Can you work these out from the model? Positions are in its coordinate system, mm. Coordinates: 2 decimals unless noted, no trailing zeros. Loops run counter-clockwise (first coordinate to the right, second up) from the corner with the lowest first, then second, coordinate; pieces in that order, holes last.
```python
from build123d import *

# Parameters (mm, degrees)
ESQUISSE1_W             = 143
ESQUISSE1_H             = 200
BOSS_EXTRU_1_DEPTH      = 6
ESQUISSE2_W             = 6
ESQUISSE2_H             = 30
ESQUISSE2_W_2           = 29
ESQUISSE2_H_2           = 6
ESQUISSE2_W_3           = 24
ENL_V_MAT_EXTRU_1_DEPTH = 6
ESQUISSE3_W             = 6
ESQUISSE3_H             = 37
BOSS_EXTRU_2_DEPTH      = 6
ESQUISSE4_W             = 36
ESQUISSE4_H             = 200
ENL_V_MAT_EXTRU_2_DEPTH = 10
ESQUISSE5_R             = 2.995
ENL_V_MAT_EXTRU_3_DEPTH = 3
ESQUISSE6_R             = 1.5
ENL_V_MAT_EXTRU_4_DEPTH = 6
ESQUISSE7_R             = 5
ENL_V_MAT_EXTRU_5_DEPTH = 10


with BuildPart() as part:
    # Esquisse1 → Boss.-Extru.1 (new body)
    with BuildSketch(Plane.XY):
        with Locations((-71.5, 100)):
            Rectangle(ESQUISSE1_W, ESQUISSE1_H)
    extrude(amount=BOSS_EXTRU_1_DEPTH)

    # Esquisse2 → Enlèv. mat.-Extru.1 (cut)
    with BuildSketch(Plane(origin=(0, 0, 0), x_dir=(-1, 0, 0), z_dir=(0, 0, -1))):
        with Locations((3, 65)):
            Rectangle(ESQUISSE2_W, ESQUISSE2_H)
        with Locations((3, 135)):
            Rectangle(ESQUISSE2_W, ESQUISSE2_H)
        with Locations((50.5, 3)):
            Rectangle(ESQUISSE2_W_2, ESQUISSE2_H_2)
        with Locations((104, 3)):
            Rectangle(ESQUISSE2_W_3, ESQUISSE2_H_2)
        with Locations((50.5, 197)):
            Rectangle(ESQUISSE2_W_2, ESQUISSE2_H_2)
        with Locations((104, 197)):
            Rectangle(ESQUISSE2_W_3, ESQUISSE2_H_2)
    extrude(amount=-ENL_V_MAT_EXTRU_1_DEPTH, mode=Mode.SUBTRACT)

    # Esquisse3 → Boss.-Extru.2 (add)
    with BuildSketch(Plane.ZY.offset(143)):
        with Locations((3, 62.5)):
            Rectangle(ESQUISSE3_W, ESQUISSE3_H)
        with Locations((3, 137.5)):
            Rectangle(ESQUISSE3_W, ESQUISSE3_H)
    extrude(amount=BOSS_EXTRU_2_DEPTH)

    # Esquisse4 → Enlèv. mat.-Extru.2 (cut)
    with BuildSketch(Plane(origin=(0, 0, 0), x_dir=(-1, 0, 0), z_dir=(0, 0, -1))):
        with Locations((18, 100)):
            Rectangle(ESQUISSE4_W, ESQUISSE4_H)
    extrude(amount=-ENL_V_MAT_EXTRU_2_DEPTH, mode=Mode.SUBTRACT)

    # Esquisse5 → Enlèv. mat.-Extru.3 (cut)
    with BuildSketch(Plane(origin=(0, 0, 0), x_dir=(-1, 0, 0), z_dir=(0, 0, -1))):
        with Locations((78.5, 3)):
            Circle(ESQUISSE5_R)
        with Locations((129.5, 3)):
            Circle(ESQUISSE5_R)
        with Locations((78.5, 197)):
            Circle(ESQUISSE5_R)
        with Locations((129.5, 197)):
            Circle(ESQUISSE5_R)
        with Locations((146, 62.5)):
            Circle(ESQUISSE5_R)
        with Locations((146, 137.5)):
            Circle(ESQUISSE5_R)
    extrude(amount=-ENL_V_MAT_EXTRU_3_DEPTH, mode=Mode.SUBTRACT)

    # Esquisse6 → Enlèv. mat.-Extru.4 (cut)
    with BuildSketch(Plane(origin=(0, 0, 0), x_dir=(-1, 0, 0), z_dir=(0, 0, -1))):
        with Locations((78.5, 3)):
            Circle(ESQUISSE6_R)
        with Locations((129.5, 3)):
            Circle(ESQUISSE6_R)
        with Locations((78.5, 197)):
            Circle(ESQUISSE6_R)
        with Locations((129.5, 197)):
            Circle(ESQUISSE6_R)
        with Locations((146, 62.5)):
            Circle(ESQUISSE6_R)
        with Locations((146, 137.5)):
            Circle(ESQUISSE6_R)
    extrude(amount=-ENL_V_MAT_EXTRU_4_DEPTH, mode=Mode.SUBTRACT)

    # Esquisse7 → Enlèv. mat.-Extru.5 (cut)
    with BuildSketch(Plane(origin=(0, 0, 0), x_dir=(-1, 0, 0), z_dir=(0, 0, -1))):
        with Locations((123, 68)):
            Circle(ESQUISSE7_R)
    extrude(amount=-ENL_V_MAT_EXTRU_5_DEPTH, mode=Mode.SUBTRACT)


solid = part.part
```
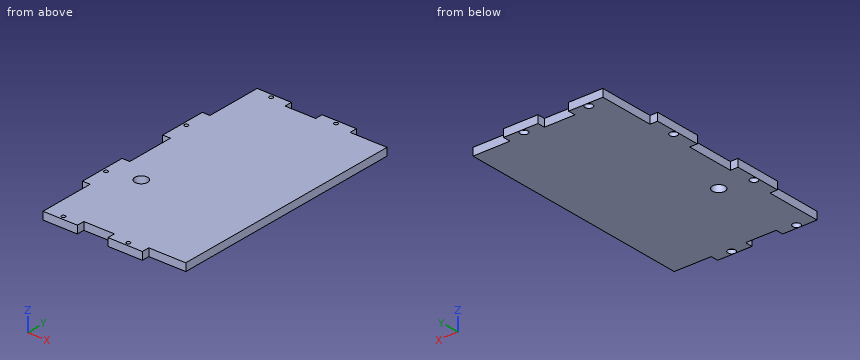
Item 1: Suppose I cut it at C-C, the plane y = 167. Please give me the cut outline in (x, z).
Results are:
outline: (-143, 0) - (-36, 0) - (-36, 6) - (-143, 6) - close
Item 2: Suppose I cut it at A-A, the plane y = 68. Please give me the cut outline in (x, z).
Results are:
outline: (-149, 0) - (-128, 0) - (-128, 6) - (-149, 6) - close; (-118, 0) - (-36, 0) - (-36, 6) - (-118, 6) - close
Item 3: Suppose I cut it at B-B, the plane x = -123. Please give me the cut outline in (y, z).
Results are:
outline: (0, 0) - (63, 0) - (63, 6) - (0, 6) - close; (73, 0) - (200, 0) - (200, 6) - (73, 6) - close
Item 4: I need wall thicknesses on line 1 along Y through (x, z) = (-78.5, 4.4); line 2 along Y through (x, z) = (-146, 3.65); line 3 along Y through (x, z) = (-77.5, 1.55). Which ranges of each line are inside material? Lowest first, please.
Results are:
line 1: y = 0 to 1.5, 4.5 to 195.5, 198.5 to 200
line 2: y = 44 to 61, 64 to 81, 119 to 136, 139 to 156
line 3: y = 0 to 0.18, 5.82 to 194.18, 199.82 to 200
Item 5: I'm going to push flat-ended pins straight in: P1, Ø1.5, axis at y = 91, z = 0.5, coming from the -X side; P2, Ø6.5, axis at x = -146.5, y = 138, coming from the -Z side; P3, Ø1.8, axis at y = 3, z = 3.5, coming from the +X side; P4, Ø1.5, axis at x = -57, z = 2, coming from the -Y side. Where does each tip first touch, or does it pass through?
Results are:
P1: stops at x = -143
P2: stops at z = 0
P3: stops at x = -65
P4: stops at y = 6
Item 6: Suppose I cut it at D-D, the plane x = -105.5. Please give me the cut outline in (y, z), plus the area to 3 significant figures.
Results are:
outline: (6, 0) - (194, 0) - (194, 6) - (6, 6) - close
area: 1,130 mm2
